Can you work these out from the model? Positions are in its coordinate system, mm. Face numbers are marked on the shaded views. A direction names the side the tool comes from. Give positions to 0.01 mm unless a question says otherwise; leave off trailing zeros. Write each loop counter-clockwise with the first axis right and the second up, starting at its lowest first coordinate (ties: lowest second). Pieces come first, ordered by that corner, then holes. Notation, with made-up numbers: M 22.25,85.5 L 31.25,85.5 A28 ccw 31.25,107.5 Z; hole C -26,-35.5 d3. An arc over 180 degrees is marked long. Write each question's results on one line, items separated by ' | '.
Autodesk Inventor part; units mm, degrees
ref_plane "YZ Plane" through (0, 0, 0) normal (1, 0, 0) x (0, 1, 0)
ref_plane "XZ Plane" through (0, 0, 0) normal (0, 1, 0) x (-1, 0, 0)
ref_plane "XY Plane" through (0, 0, 0) normal (0, 0, 1) x (1, 0, 0)
sketch "Sketch1" plane through (0, 0, 0) normal (0, 1, 0) x (-1, 0, 0)
  line L0 (-12.7, 25.4) -> (12.7, 25.4)
  line L1 (12.7, 25.4) -> (12.7, -25.4)
  line L2 (12.7, -25.4) -> (-12.7, -25.4)
  line L3 (-12.7, -25.4) -> (-12.7, 25.4)
  line L4 (-12.7, 25.4) -> (12.7, -25.4) construction
  line L5 (12.7, 25.4) -> (-12.7, -25.4) construction
  line L6 (11.1125, 23.8125) -> (-11.1125, 23.8125)
  line L7 (-11.1125, 23.8125) -> (-11.1125, -23.8125)
  line L8 (-11.1125, -23.8125) -> (11.1125, -23.8125)
  line L9 (11.1125, -23.8125) -> (11.1125, 23.8125)
  line L10 (11.1125, 23.8125) -> (-11.1125, -23.8125) construction
  line L11 (-11.1125, 23.8125) -> (11.1125, -23.8125) construction
  point P0 (0, 0)
  dimension "d0" = 25.4
  dimension "d1" = 50.8
  dimension "d2" = 22.225
  dimension "d3" = 47.625
extrude "Extrusion1" add sketch "Sketch1" along normal blind 279.4
sketch "Sketch2" plane through (12.7, 0, 25.4) normal (1, 0, 0) x (0, 0, -1)
  line L0 (0, 279.4) -> (50.8, 279.4)
  line L1 (0, 0) -> (0, 279.4)
  point P0 (25.4, 0)
  point P1 (25.4, 190.5)
  dimension "d21" = 25.4
  dimension "d24" = 190.5
hole "Hole1" at (12.7, 190.5, 0) direction (-1, 0, 0) diameter 28.575 end through all
sketch "Sketch3" plane through (12.7, 0, 25.4) normal (1, 0, 0) x (0, 0, -1)
  line L0 (50.8, 0) -> (50.8, 279.4)
  line L1 (0, 0) -> (50.8, 0)
  point P0 (25.4, 0)
  point P1 (25.4, 25.4)
  dimension "d22" = 25.4
  dimension "d23" = 25.4
hole "Hole2" at (12.7, 25.4, 0) direction (-1, 0, 0) diameter 28.575 end through all
sketch "Sketch5" plane through (12.7, 0, 25.4) normal (1, 0, 0) x (0, 0, -1)
  line L0 (25.4, 254) -> (25.4, 246.38) construction
  line L1 (17.78, 254) -> (17.78, 246.38)
  line L2 (33.02, 246.38) -> (33.02, 254)
  arc A0 (33.02, 254) -> (17.78, 254) centre (25.4, 254) ccw
  arc A1 (17.78, 246.38) -> (33.02, 246.38) centre (25.4, 246.38) ccw
  line L3 (0, 279.4) -> (50.8, 279.4)
  point P0 (25.4, 0)
  point P1 (25.4, 250.19)
  dimension "d34" = 7.62
  dimension "d35" = 15.24
  dimension "d36" = 25.4
extrude "Extrusion2" cut sketch "Sketch5" against normal through all
sketch "Sketch6" plane through (12.7, 0, 25.4) normal (1, 0, 0) x (0, 0, -1)
  line L0 (7.5819, 268.7054) -> (43.2181, 268.7054) construction
  line L1 (43.2181, 268.7054) -> (43.2181, 233.0692) construction
  line L2 (43.2181, 233.0692) -> (7.5819, 233.0692) construction
  line L3 (7.5819, 233.0692) -> (7.5819, 268.7054) construction
  line L4 (7.5819, 268.7054) -> (43.2181, 233.0692) construction
  line L5 (43.2181, 268.7054) -> (7.5819, 233.0692) construction
  line L6 (7.5819, 268.7054) -> (7.5819, 261.0854) construction
  line L7 (4.8514, 268.7054) -> (4.8514, 261.0854)
  line L8 (10.3124, 261.0854) -> (10.3124, 268.7054)
  arc A0 (10.3124, 268.7054) -> (4.8514, 268.7054) centre (7.5819, 268.7054) ccw
  arc A1 (4.8514, 261.0854) -> (10.3124, 261.0854) centre (7.5819, 261.0854) ccw
  line L9 (43.2181, 233.0692) -> (43.2181, 240.6892) construction
  line L10 (45.9486, 233.0692) -> (45.9486, 240.6892)
  line L11 (40.4876, 240.6892) -> (40.4876, 233.0692)
  arc A2 (40.4876, 233.0692) -> (45.9486, 233.0692) centre (43.2181, 233.0692) ccw
  arc A3 (45.9486, 240.6892) -> (40.4876, 240.6892) centre (43.2181, 240.6892) ccw
  point P0 (25.4, 0)
  point P1 (25.4, 250.8873)
  point P2 (7.5819, 264.8954)
  point P3 (43.2181, 236.8792)
  dimension "d39" = 35.6362
  dimension "d40" = 35.6362
  dimension "d46" = 7.62
  dimension "d47" = 5.461
  dimension "d48" = 7.62
  dimension "d49" = 5.461
extrude "Extrusion3" cut sketch "Sketch6" against normal through all
sketch "Sketch7" plane through (-12.7, 0, -25.4) normal (-1, 0, 0) x (0, 0, 1)
  arc A0 (10.3124, 240.6892) -> (4.8514, 240.6892) centre (7.5819, 240.6892) ccw
  line L0 (7.5819, 240.6892) -> (7.5819, 232.5183) construction
  line L1 (3.1369, 240.6892) -> (3.1369, 232.5183)
  line L2 (12.0269, 232.5183) -> (12.0269, 240.6892)
  arc A1 (12.0269, 240.6892) -> (3.1369, 240.6892) centre (7.5819, 240.6892) ccw
  arc A2 (3.1369, 232.5183) -> (12.0269, 232.5183) centre (7.5819, 232.5183) ccw
  arc A3 (45.9486, 268.7054) -> (40.4876, 268.7054) centre (43.2181, 268.7054) ccw
  arc A4 (40.4876, 261.0854) -> (45.9486, 261.0854) centre (43.2181, 261.0854) ccw
  line L3 (43.2181, 268.7054) -> (43.2181, 261.0854) construction
  line L4 (38.7731, 268.7054) -> (38.7731, 261.0854)
  line L5 (47.6631, 261.0854) -> (47.6631, 268.7054)
  arc A5 (47.6631, 268.7054) -> (38.7731, 268.7054) centre (43.2181, 268.7054) ccw
  arc A6 (38.7731, 261.0854) -> (47.6631, 261.0854) centre (43.2181, 261.0854) ccw
  point P0 (25.4, 0)
  point P1 (7.5819, 236.6038)
  point P2 (43.2181, 264.8954)
  dimension "d50" = 8.89
  dimension "d51" = 8.89
extrude "Extrusion4" cut sketch "Sketch7" against normal blind 12.7
properties part number "2x1 Front with motor mount" material "Aluminum 6061"
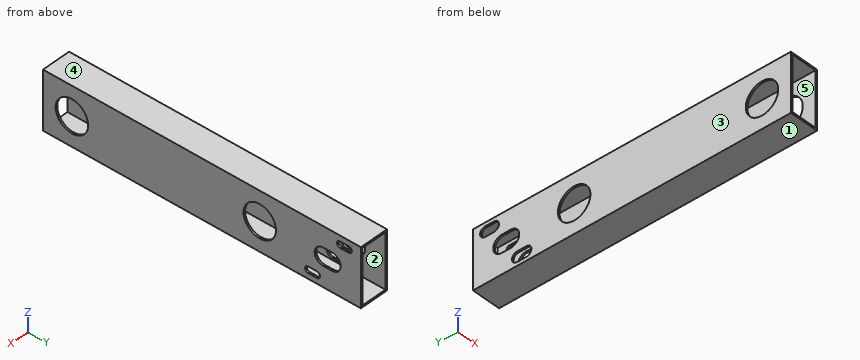
Item 1: If I drill on line 1 (Y direction, x = 11.55, z = 0); line 2 (X direction, y = 261, z = -11); line 3 (Z direction, x = -11.5, y = 190.5), over which ranges is the centre line in solid material (lowest first)? Write a range as from..to.
Geometry says:
line 1: y = 0..11.11, 39.69..176.21, 204.79..238.76, 261.62..279.4 | line 2: x = -12.7..-11.11, 11.11..12.7 | line 3: z = -25.4..-14.29, 14.29..25.4
Item 2: I want a section at A-A, the plane y = 190.5. Please give me the cut outline in (x, z).
Geometry says:
outline: M -12.7,-25.4 L 12.7,-25.4 L 12.7,-14.29 L 11.11,-14.29 L 11.11,-23.81 L -11.11,-23.81 L -11.11,-14.29 L -12.7,-14.29 Z; M -12.7,14.29 L -11.11,14.29 L -11.11,23.81 L 11.11,23.81 L 11.11,14.29 L 12.7,14.29 L 12.7,25.4 L -12.7,25.4 Z
Item 3: I want a section at D-D, the plane x = -4.75. Please give me the cut outline in (y, z), and give its area (3 significant figures).
Geometry says:
outline: M 0,-25.4 L 279.4,-25.4 L 279.4,-23.81 L 0,-23.81 Z; M 0,23.81 L 279.4,23.81 L 279.4,25.4 L 0,25.4 Z | area: 887 mm2
Item 4: For the marked faces 1 and 2, which set-ups out of +Z, -Z, +X, -X, +Y, -Y let a thin tool reach every point of the face, with its end or its side?
Geometry says:
face 1: -Z, +X, -X, +Y, -Y | face 2: +Y, -Y
Item 5: Thinking about a two-plate mould opening in X: for the marked faces 3, 4 and 5, which applies, +X half, -X half, draft (parallel to the pull), parting line (faces both ways), or undercut?
Geometry says:
face 3: -X half | face 4: draft | face 5: undercut
Item 6: I want a section at B-B, the plane z = 0. Give the number of separate pieces and of enclosed holes in the cut face, and give its area (3 significant figures).
Geometry says:
separate pieces: 8 | enclosed holes: 0 | area: 633 mm2
Item 7: I'm going to push a flat-ended pin straight in: pin 1 (17 mm diameter, centred on y = 190.5, z = 0, fed in from +X) (3 decimals). Where does the tip first touch, or does it pass through?
Geometry says:
pin 1: passes through
Item 8: I want a section at C-C, the plane y = 57. Please give me the cut outline in (x, z), and give its area (3 significant figures).
Geometry says:
outline: M -12.7,-25.4 L 12.7,-25.4 L 12.7,25.4 L -12.7,25.4 Z; hole M -11.11,-23.81 L 11.11,-23.81 L 11.11,23.81 L -11.11,23.81 Z | area: 232 mm2
